Can you work these out from the model? Positions are in its coordinate system, mm. Face numbers are marked on the shaded views. A direction names the side the tool comes from. Coordinates: 2 decimals unless noted, no trailing zeros. Order: outer loops, then holes, each group sorted by start corner. A loop starts at its lowest first (then second) coordinate and runs counter-clockwise, first axis right, second up. Notation, with made-up numbers: (-19, 75.5) -> (32, 75.5) arc R12 ccw to (32, 90.5) -> close; hole circle Ø3 at (27.5, 79.5). An arc over 180 degrees is marked (long way). Answer in a Markdown table with one row per item.
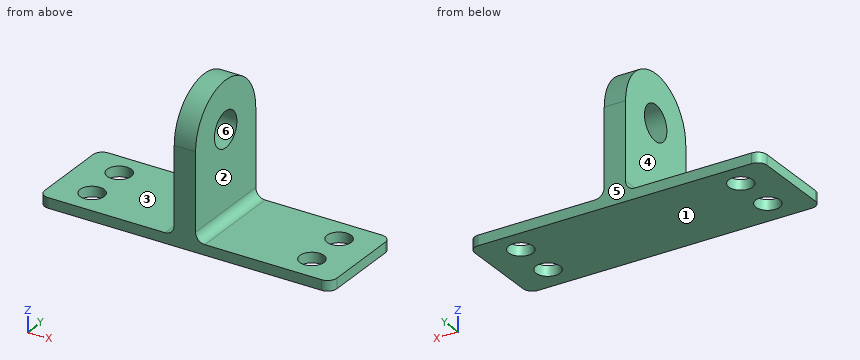
```python
from build123d import *

# Parameters (mm, degrees)
SKETCH1_R             = 3.302
BOSS_EXTRUDE1_DEPTH   = 2.794
SKETCH1_W             = 37.084
SKETCH1_H             = 25.908
BOSS_EXTRUDE1_2_DEPTH = 2.794
SKETCH1_7_W           = 5.842
SKETCH1_7_H           = 25.908
BOSS_EXTRUDE2_DEPTH   = 39.624
FILLET1_R             = 2.54
SKETCH2_R             = 4.826
CUT_EXTRUDE4_DEPTH    = 39.624
CUT_EXTRUDE5_DEPTH    = 39.624
FILLET2_R             = 2.54


with BuildPart() as part:
    # Sketch1 → Boss-Extrude1 (new body)
    with BuildSketch(Plane.XY):
        Polygon((-0.948051948, -5.19147622), (-0.948051948, -25.336571429), (36.135948052, -25.336571429), (36.135948052, 0.571428571), (8.957948052, 0.571428571), (-0.948051948, 0.571428571), align=None)
        with Locations((8.957948052, -17.970571429)):
            Circle(SKETCH1_R, mode=Mode.SUBTRACT)
        with Locations((8.957948052, -6.286571429)):
            Circle(SKETCH1_R, mode=Mode.SUBTRACT)
    extrude(amount=BOSS_EXTRUDE1_DEPTH)



with BuildPart() as body_2:
    # Sketch1 → Boss-Extrude1 2 (new body)
    with BuildSketch(Plane.XY):
        with Locations((60.519948052, -12.382571429)):
            Rectangle(SKETCH1_W, SKETCH1_H)
        with Locations((69.155948052, -17.970571429)):
            Circle(SKETCH1_R, mode=Mode.SUBTRACT)
        with Locations((69.155948052, -6.286571429)):
            Circle(SKETCH1_R, mode=Mode.SUBTRACT)
    extrude(amount=BOSS_EXTRUDE1_2_DEPTH)


with BuildPart() as part_1:
    add(part.part)

    add(body_2.part)  # Boss-Extrude2 merges body 2
    # Sketch1_7 → Boss-Extrude2 (add)
    with BuildSketch(Plane.XY):
        with Locations((39.056948052, -12.382571429)):
            Rectangle(SKETCH1_7_W, SKETCH1_7_H)
    extrude(amount=BOSS_EXTRUDE2_DEPTH)

    # Fillet1
    fillet1_edges = [part_1.edges().sort_by_distance(p)[0] for p in [
        (-0.948051948, -25.336571429, 1.397),
        (-0.948051948, 0.571428571, 1.397),
        (79.061948052, 0.571428571, 1.397),
        (79.061948052, -25.336571429, 1.397),
    ]]
    fillet(fillet1_edges, radius=FILLET1_R)

    # Sketch2 → Cut-Extrude4 (cut)
    with BuildSketch(Plane(origin=(41.977948052, 0, 0), x_dir=(0, 0, -1), z_dir=(1, 0, 0))):
        with Locations((-26.416, -12.382571429)):
            Circle(SKETCH2_R)
    extrude(amount=-CUT_EXTRUDE4_DEPTH, mode=Mode.SUBTRACT)

    # Sketch2_11 → Cut-Extrude5 (cut)
    with BuildSketch(Plane(origin=(41.977948052, 0, 0), x_dir=(0, 0, -1), z_dir=(1, 0, 0))):
        with BuildLine():
            ThreePointArc((-26.416, -25.336571429), (-39.37, -12.382571429), (-26.416, 0.571428571))
            Line((-26.416, 0.571428571), (-39.624, 0.571428571))
            Line((-39.624, 0.571428571), (-39.624, -25.336571429))
            Line((-39.624, -25.336571429), (-26.416, -25.336571429))
        make_face()
    extrude(amount=-CUT_EXTRUDE5_DEPTH, mode=Mode.SUBTRACT)

    # Fillet2
    fillet2_edges = [part_1.edges().sort_by_distance(p)[0] for p in [
        (41.977948052, -12.382571429, 2.794),
        (36.135948052, -12.382571429, 2.794),
    ]]
    fillet(fillet2_edges, radius=FILLET2_R)


solid = part_1.part
```
(1) Suppose I cut it at D-D (y = -16). Please give me the cut outline in (x, z), and give its area (3 significant figures).
Response values:
| item | result |
|---|---|
| outline | (-0.95, 0) -> (6.31, 0) -> (6.31, 2.79) -> (-0.95, 2.79) -> close; (11.61, 0) -> (66.51, 0) -> (66.51, 2.79) -> (44.52, 2.79) arc R2.54 cw to (41.98, 5.33) -> (41.98, 23.22) -> (36.14, 23.22) -> (36.14, 5.33) arc R2.54 cw to (33.6, 2.79) -> (11.61, 2.79) -> close; (36.14, 29.61) -> (41.98, 29.61) -> (41.98, 38.85) -> (36.14, 38.85) -> close; (71.81, 0) -> (79.06, 0) -> (79.06, 2.79) -> (71.81, 2.79) -> close |
| area | 370 mm2 |
(2) I need wall thicknesses on line 1 (Z direction, x = 9.5, y = -12); line 2 (X direction, y = -7.5, z = 35.5); line 3 (Y direction, x = 37, z = 30). Which ranges of each line are inside material? Lowest first, please. Write a range as [from, to].
Response values:
| item | result |
|---|---|
| line 1 | [0, 2.79] |
| line 2 | [36.14, 41.98] |
| line 3 | [-24.83, -15.61], [-9.15, 0.07] |
(3) Suppose I cut it at C-C (x = 29). Please give me the cut outline in (y, z), and give its area (3 significant figures).
Response values:
| item | result |
|---|---|
| outline | (-25.34, 0) -> (0.57, 0) -> (0.57, 2.79) -> (-25.34, 2.79) -> close |
| area | 72.4 mm2 |
(4) Suppose I cut it at A-A (y = -5.25). Please give me the cut outline in (x, z), and give its area (3 significant figures).
Response values:
| item | result |
|---|---|
| outline | (-0.95, 0) -> (5.82, 0) -> (5.82, 2.79) -> (-0.95, 2.79) -> close; (12.09, 0) -> (66.02, 0) -> (66.02, 2.79) -> (44.52, 2.79) arc R2.54 cw to (41.98, 5.33) -> (41.98, 37.23) -> (36.14, 37.23) -> (36.14, 5.33) arc R2.54 cw to (33.6, 2.79) -> (12.09, 2.79) -> close; (72.29, 0) -> (79.06, 0) -> (79.06, 2.79) -> (72.29, 2.79) -> close |
| area | 392 mm2 |
(5) Will these pins go through, and if not, where does the flat tip stop? pin 1 Ø13 at (y, z) = (-12.5, 28) entering from +X; pin 2 Ø10 at (y, z) = (-17, 34.5) entering from -X; pin 3 Ø4 at (x, y) = (10.5, -9.5) entering from +Z.
Response values:
| item | result |
|---|---|
| pin 1 | x = 41.98 |
| pin 2 | x = 36.14 |
| pin 3 | z = 2.79 |
(6) We'd pull the mould along Y, two halves only. Please class the marked faces 4, 5 and 6: +Y half, -Y half, draft (parallel to the pull), parting line (faces both ways), or undercut.
Response values:
| item | result |
|---|---|
| face 4 | draft |
| face 5 | +Y half |
| face 6 | undercut |
(7) Suppose I cut it at B-B (y = -10.5). Please give me the cut outline in (x, z).
Response values:
| item | result |
|---|---|
| outline | (-0.95, 0) -> (79.06, 0) -> (79.06, 2.79) -> (44.52, 2.79) arc R2.54 cw to (41.98, 5.33) -> (41.98, 21.97) -> (36.14, 21.97) -> (36.14, 5.33) arc R2.54 cw to (33.6, 2.79) -> (-0.95, 2.79) -> close; (36.14, 30.86) -> (41.98, 30.86) -> (41.98, 39.23) -> (36.14, 39.23) -> close |
(8) On a 3-axis mill with a long thin cutter (end or side, diameter ignored), from which of +Z, -Z, +X, -X, +Y, -Y can I reach the whole of each face in a straight line? I mean the marked faces 1, 2 and 3. Say none if no direction works.
Response values:
| item | result |
|---|---|
| face 1 | -Z, +X, -X, +Y, -Y |
| face 2 | +Z, +X, +Y, -Y |
| face 3 | +Z, -X, +Y, -Y |
